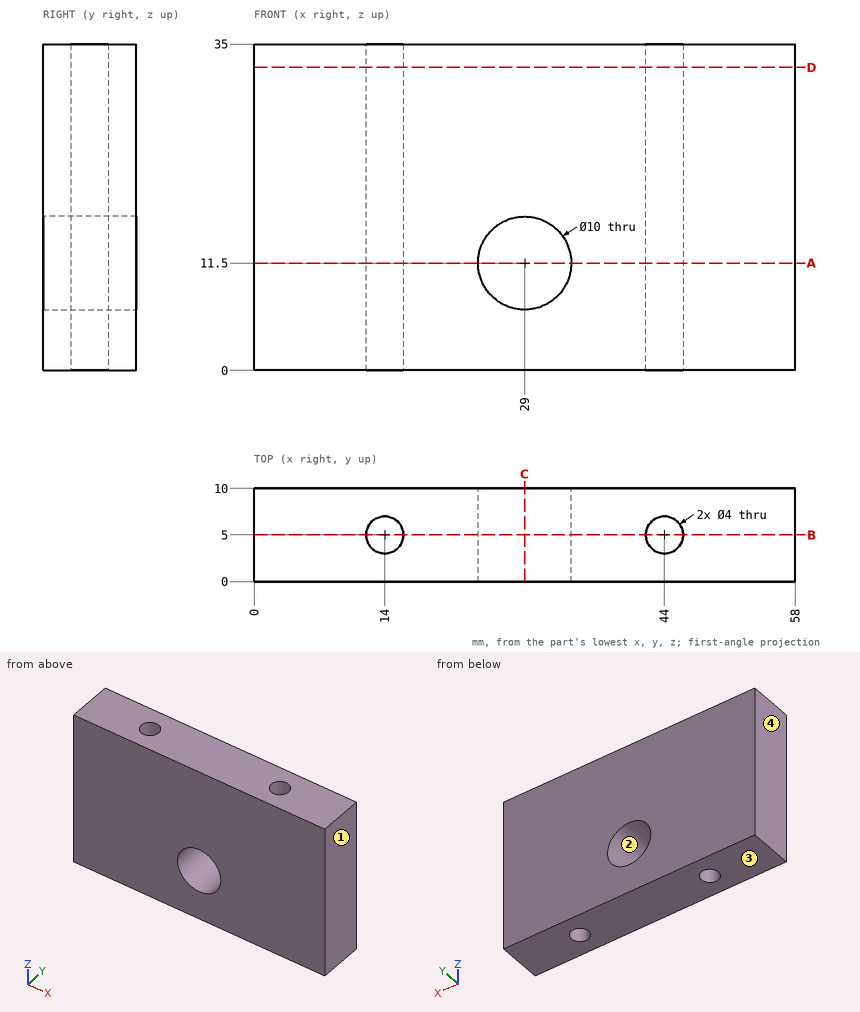
Verification items for this drawing (mm, ordinates from the low corner). Coordinates: 2 decimals unless noted, no trailing zeros. Loops run counter-clockwise (first coordinate to the right, second up) from the corner with the lowest first, then second, coordinate; pieces in that order, holes last. Notation, with made-up numbers: (50.25, 33) - (98.25, 33) arc R6 ccw to (98.25, 44) - close; hole circle Ø6 at (-36.75, -40). An arc over 180 degrees is marked (long way). Use one line per item in the form item = value. Start each with the question number.
Item 1: Section check C-C, the plane x = 29. Enter the section's corners in (y, z), and give its area (3 significant figures).
Item 2: Thickness scan on probe 1 along X at (y, z) = (6, 11.5); probe 2 along X at (y, z) = (3.25, 11.5); probe 3 along X at (y, z) = (5, 18). Record the ranges inside material, lowest first.
Item 3: Section check A-A, the plane z = 11.5. Enter the section's corners in (x, y), and give its area (3 significant figures).
Item 4: Section check D-D, the plane z = 32.5. Enter the section's corners in (x, y).
Item 5: Gauge pin test, flat end, axial feed: pin 1 (9 mm diameter, centred on x = 29, z = 11.5, fed in from +Y). Record the tip position at first contact, or that the pin passes through.
Item 6: Mould release check, pull along X, two halves, no side actions. Record for the marked faces 1, 2, 3 and 4: +X half, -X half, draft (parallel to the pull), parting line (faces both ways), or undercut.
Item 7: Section check B-B, the plane y = 5. Enter the section's corners in (x, z), and give its area (3 significant figures).
Computed:
q1.outline = (0, 0) - (10, 0) - (10, 6.5) - (0, 6.5) - close; (0, 16.5) - (10, 16.5) - (10, 35) - (0, 35) - close
q1.area = 250 mm2
q2.probe_1 = 0 to 12.27, 15.73 to 24, 34 to 42.27, 45.73 to 58
q2.probe_2 = 0 to 13.03, 14.97 to 24, 34 to 43.03, 44.97 to 58
q2.probe_3 = 0 to 12, 16 to 42, 46 to 58
q3.outline = (0, 0) - (24, 0) - (24, 10) - (0, 10) - close; (34, 0) - (58, 0) - (58, 10) - (34, 10) - close; hole circle Ø4 at (14, 5); hole circle Ø4 at (44, 5)
q3.area = 455 mm2
q4.outline = (0, 0) - (58, 0) - (58, 10) - (0, 10) - close; hole circle Ø4 at (14, 5); hole circle Ø4 at (44, 5)
q5.pin_1 = through
q6.face_1 = +X half
q6.face_2 = undercut
q6.face_3 = draft
q6.face_4 = -X half
q7.outline = (0, 0) - (12, 0) - (12, 35) - (0, 35) - close; (16, 0) - (42, 0) - (42, 35) - (16, 35) - close; (46, 0) - (58, 0) - (58, 35) - (46, 35) - close; hole circle Ø10 at (29, 11.5)
q7.area = 1,670 mm2
